The listing builds one solid part. Answer for the finished solid, in the listing's coordinates (mm). Face numbers are marked on the shaded views. A direction names the side the tool comes from. Coordinates: 2 decimals unless noted, no trailing zeros. Loops run counter-clockwise (first coordinate to the right, second up) from the corner with the lowest first, then second, coordinate; pieces in that order, holes last. Notation, with made-up numbers: (12.5, -16) - (69.5, -16) arc R29 ccw to (69.5, 5) - close; hole circle Ø1 at (-12.75, 7). An arc over 180 degrees is marked (long way). One line per question, with ' | ' between items.
from build123d import *

# Parameters (mm, degrees)
SKETCH1_R                = 52.508103221
BOSS_EXTRUDE1_DEPTH      = 36.322
FILLET1_R                = 10.16
SHELL1_T                 = -5.08
CUT_EXTRUDE1_DEPTH       = 8.89
LPATTERN1_COUNT          = 7
LPATTERN1_PITCH          = 8.89
BOSS_EXTRUDE2_DEPTH      = 7.112
BOSS_EXTRUDE2_DEPTH_BACK = 5.08
SKETCH6_R                = 22.438749527
SKETCH6_R_2              = 11.562158197
FILLET2_R                = 2.54
SKETCH7_R                = 6.688781748
BOSS_EXTRUDE3_DEPTH      = 7.62
CIRPATTERN4_COUNT        = 3


with BuildPart() as part:
    # Sketch1 → Boss-Extrude1 (new body)
    with BuildSketch(Plane(origin=(0, 0, 0), x_dir=(0, 0, -1), z_dir=(1, 0, 0))):
        with Locations((1.26107084, 0)):
            Circle(SKETCH1_R)
    extrude(amount=BOSS_EXTRUDE1_DEPTH)

    # Fillet1
    fillet1_edges = [part.edges().sort_by_distance(p)[0] for p in [
        (36.322, 0, 51.247032381),
    ]]
    fillet(fillet1_edges, radius=FILLET1_R)

    # Shell1
    shell1_openings = [part.faces().sort_by_distance(p)[0] for p in [
        (0, 0, -1.26107084),
    ]]
    offset(amount=SHELL1_T, openings=shell1_openings, kind=Kind.INTERSECTION)

    # Sketch2 → Cut-Extrude1 (cut)
    with BuildSketch(Plane(origin=(36.322, 0, 0), x_dir=(0, 0, -1), z_dir=(1, 0, 0))):
        with BuildLine():
            Line((-34.904419589, 11.386418641), (-17.571533949, -31.67067029))
            ThreePointArc((-17.571533949, -31.67067029), (-18.64799848, -34.197771514), (-21.175099704, -33.121306983))
            Line((-21.175099704, -33.121306983), (-38.507985344, 9.935781948))
            ThreePointArc((-38.507985344, 9.935781948), (-37.431520813, 12.462883172), (-34.904419589, 11.386418641))
        make_face()
    cut_extrude1 = extrude(amount=-CUT_EXTRUDE1_DEPTH, mode=Mode.SUBTRACT)

    # LPattern1: Cut-Extrude1 ×7
    with Locations(*[Vector(0, 0.5493346615269119, -0.8356024351598751) * (i * LPATTERN1_PITCH) for i in range(1, LPATTERN1_COUNT)]):
        add(cut_extrude1, mode=Mode.SUBTRACT)

    # Sketch6 → Boss-Extrude2 (add, two sides: drawn at the far end of the back side and taken through both)
    with BuildSketch(Plane(origin=(36.322, 0, 0), x_dir=(0, 0, -1), z_dir=(1, 0, 0)).offset(-BOSS_EXTRUDE2_DEPTH_BACK)):
        Circle(SKETCH6_R)
        Circle(SKETCH6_R_2, mode=Mode.SUBTRACT)
    extrude(amount=BOSS_EXTRUDE2_DEPTH + BOSS_EXTRUDE2_DEPTH_BACK)

    # Fillet2
    fillet2_edges = [part.edges().sort_by_distance(p)[0] for p in [
        (43.434, 0, 22.438749527),
    ]]
    fillet(fillet2_edges, radius=FILLET2_R)

    # Sketch7 → Boss-Extrude3 (add)
    with BuildSketch(Plane.ZY):
        with BuildLine():
            Line((-68.934787108, 24.910674724), (-51.515117818, 15.21945026))
            Line((-51.515117818, 15.21945026), (-42.107991595, 32.994392988))
            Line((-42.107991595, 32.994392988), (-58.035685788, 42.734194788))
            ThreePointArc((-58.035685788, 42.734194788), (-72.771352602, 39.50090458), (-68.934787108, 24.910674724))
        make_face()
        with Locations((-63.852046762, 34.04673965)):
            Circle(SKETCH7_R, mode=Mode.SUBTRACT)
    boss_extrude3 = extrude(amount=-BOSS_EXTRUDE3_DEPTH)

    # CirPattern4: Boss-Extrude3 ×3 about axis
    cirpattern4_axis = Axis((0, 0, -1.26107084), (1, 0, 0))
    for i in range(1, CIRPATTERN4_COUNT):
        add(boss_extrude3.rotate(cirpattern4_axis, i * 360 / CIRPATTERN4_COUNT))


solid = part.part
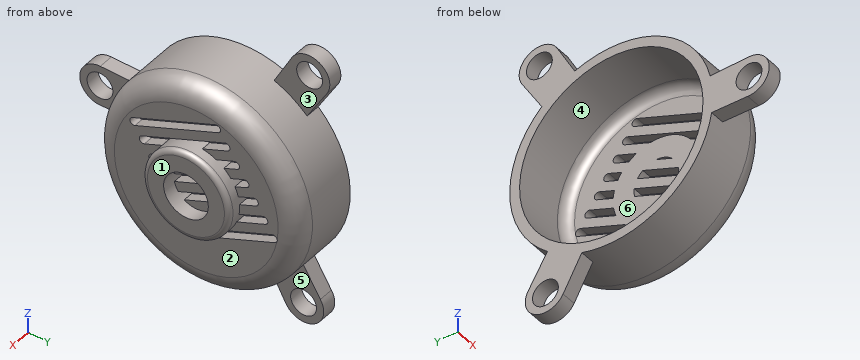
Item 1: Which of the six approach directions +Z, -Z, +X, -X, +Y, -Y give full straight-line access (tool end or side, diameter ignored) to the marked faces 1, 2 and 3?
Taken from the geometry:
face 1: +Z, -Z, +X, +Y, -Y | face 2: +X | face 3: +Z, +X, +Y
Item 2: Find the intervals of material crossed by line 1 (Z direction, x = 4, y = 31); line 2 (Z direction, x = 13, y = 0); line 3 (Z direction, x = 7.5, y = 38.5), in increasing order. Write a range as [from, to].
Taken from the geometry:
line 1: z = [-73.85, -69.81], [-57.9, -37.16], [34.63, 56.97], [62.07, 67.95] | line 2: z = [-53.77, -48.69], [46.17, 51.25] | line 3: z = [-73.31, -68.84], [-58.86, -51.11], [-36.97, -28.96], [26.44, 34.44], [41.37, 52.96], [66.08, 69.89]
Item 3: The mould has two halves that part along Y. Classify the marked faces 4, 5 and 6: pulls with the +Y half, pulls with the -Y half, needs draft (parallel to the pull), parting line crosses it, or undercut.
Taken from the geometry:
face 4: undercut | face 5: needs draft | face 6: undercut
Item 4: Find section A-A, the plane x = 11.5. Write down the section's boundary in (y, z), plus the area to 3 significant figures.
Taken from the geometry:
outline: circle Ø105.02 at (0, -1.26); hole circle Ø94.86 at (0, -1.26) | area: 1,590 mm2
Item 5: Each of these flat-tipped pins is pushed along its axis until it touches: pin 1 Ø5 at (y, z) = (-27, -40.5) entering from +X; pin 2 Ø6 at (x, y) = (36.5, 24.5) entering from -Z; pin 3 Ø14.5 at (y, z) = (29.5, -66) entering from +X; pin 4 Ø8 at (y, z) = (-8, 45) entering from -X. Where does it stop, or does it pass through?
Taken from the geometry:
pin 1: stops at x = 35.93 | pin 2: stops at z = -44.49 | pin 3: stops at x = 7.62 | pin 4: stops at x = 0
